The model under review builds one solid part; all positions refer to its coordinate system, in mm. A direction names the side the tool comes from. Round coordinates to 2 decimals unless told otherwise and drop trailing zeros. Order: outer loops, then holes, each group sorted by start corner. A loop starts at its lowest first (then second) coordinate and runs counter-clockwise, first axis right, second up. Notation, with made-up numbers: (52.25, -0.75) -> (70.25, -0.75) arc R14 cw to (70.25, 7.25) -> close; hole circle Ø8 at (-33, -0.75). An arc over 180 degrees is marked (long way). Use a Markdown table: item, result. Add a question column.
```python
from build123d import *

# Parameters (mm, degrees)
SKETCH1_R           = 3.175
REVOLVE1_ANGLE      = 340
SKETCH2_R           = 0.409575
BOSS_EXTRUDE1_DEPTH = 35.56
CIRPATTERN1_COUNT   = 8
SKETCH7_R           = 3.175
BOSS_EXTRUDE2_DEPTH = 17.653
SKETCH10_R          = 3.175
BOSS_EXTRUDE3_DEPTH = 50.8


with BuildPart() as part:
    # Sketch1 → Revolve1 (revolve)
    with BuildSketch(Plane.XY):
        with Locations((-34.925, 0)):
            Circle(SKETCH1_R)
    revolve(axis=Axis((0, 0, 0), (0, 1, 0)), revolution_arc=REVOLVE1_ANGLE)

    # Sketch2 → Boss-Extrude1 (add)
    with BuildSketch(Plane(origin=(0, 0, 0), x_dir=(1, 0, 0), z_dir=(0, 1, 0))):
        with Locations(Location((-29.697367501, 18.379934399, 0), (0, 0, 135.804217831))):
            Circle(SKETCH2_R)
    boss_extrude1 = extrude(amount=BOSS_EXTRUDE1_DEPTH)

    # CirPattern1: Boss-Extrude1 ×8 about axis
    cirpattern1_axis = Axis((0, 0, 0), (0, 1, 0))
    for i in range(1, CIRPATTERN1_COUNT):
        add(boss_extrude1.rotate(cirpattern1_axis, i * 360 / CIRPATTERN1_COUNT))

    # Sketch7 → Boss-Extrude2 (add)
    with BuildSketch(Plane(origin=(-34.925, 0, 0), x_dir=(0, 1, 0), z_dir=(-1, 0, 0))):
        with Locations(Location((0, 0, 0), (0, 0, 180))):
            Circle(SKETCH7_R)
    extrude(amount=BOSS_EXTRUDE2_DEPTH)

    # Sketch10 → Boss-Extrude3 (add)
    with BuildSketch(Plane(origin=(0, 0, 0), x_dir=(0, 0, -1), z_dir=(0, 1, 0))):
        with Locations(Location((0, 52.578, 0), (0, 0, 180))):
            Circle(SKETCH10_R)
    extrude(amount=-BOSS_EXTRUDE3_DEPTH)


solid = part.part
```
Q1. Wall thickness on line 1 (Y direction, x = 20, z = 31); line 2 (Y direction, x = -23, z = -30): over which ranges is each line inside the solid? List them lowest first. Write a range as [from, to].
Q2. Mouldability with a two-part tool opening along X and no side actions: class faces 1 (the flat face through (-34, 0, 0)), 2 (the flat face through (-32.86, 0.04, -11.96)), 3 (the flat face through (-53, -50.8, 0)), 4 (the cylindrical face through (-43.63, 2.52, -1.93)) as pulls with the +X half, pulls with the -X half, needs draft (parallel to the pull), parting line crosses it, or undercut.
Q3. Add section A-A (y = 16). Write out the cut boundary in (x, z).
Q4. Insertion check: pin 1 (1 mm diameter, centred on x = -54, z = -0.5, fed in from +Y); pin 2 (8 mm diameter, centred on x = 3.5, y = 6.5, fed in from -Z); pin 3 (1.5 mm diameter, centred on x = -23, y = -4, fed in from +Z); pin 4 (1.6 mm diameter, centred on x = -33.5, y = 0.5, fed in from -Z). Each pin has a flat end and moves straight along its axis. Give the tip position at first contact, or say it passes through.
Q5. Machinability: for faces 5 (the flat face through (-52.578, 1, 0)), 6 (the cylindrical face through (-55.677, -25.044, -0.688)), 7 (the flat face through (-34.925, 0, -1)), which of the approach directions +Z, -Z, +X, -X, +Y, -Y give a long, thin tool a straight path to every point of the face, cutting with its end or side? Answer none if there is none.
Q6. Add section C-C (y = -38.5). Write out the cut boundary in (x, z) (3 decimals).
Q7. Add section B-B (x = -46). Write out the cut boundary in (y, z) (3 decimals), then the cut area to 3 significant figures.
Report:
| question | item | result |
|---|---|---|
| 1 | line 1 | y = [-2.49, 2.49] |
| 1 | line 2 | y = [-1.34, 1.34] |
| 2 | face 1 | undercut |
| 2 | face 2 | pulls with the -X half |
| 2 | face 3 | needs draft |
| 2 | face 4 | undercut |
| 3 | outline | circle Ø0.82 at (-34, 8); circle Ø0.82 at (-29.7, -18.38); circle Ø0.82 at (-18.38, 29.7); circle Ø0.82 at (-8, -34); circle Ø0.82 at (8, 34); circle Ø0.82 at (18.38, -29.7); circle Ø0.82 at (29.7, 18.38); circle Ø0.82 at (34, -8) |
| 4 | pin 1 | stops at y = 0 |
| 4 | pin 2 | stops at z = -36.73 |
| 4 | pin 3 | passes through |
| 4 | pin 4 | stops at z = -19.49 |
| 5 | face 5 | +Z, -Z, -X, +Y |
| 5 | face 6 | -Y |
| 5 | face 7 | +Y, -Y |
| 6 | outline | circle Ø6.35 at (-52.578, 0) |
| 7 | outline | circle Ø6.35 at (0, 0) |
| 7 | area | 31.7 mm² |
